```python
from build123d import *

# Parameters (mm, degrees)
SKETCH1_W           = 25.4
SKETCH1_H           = 25.4
SKETCH1_W_2         = 22.225
SKETCH1_H_2         = 22.225
BOSS_EXTRUDE1_DEPTH = 501.65
SKETCH4_R           = 6.35
CUT_EXTRUDE1_DEPTH  = 26.4
SKETCH5_R           = 1.5875
CUT_EXTRUDE2_DEPTH  = 26.4
SKETCH7_R           = 3.96875
CUT_EXTRUDE3_DEPTH  = 1.5875


with BuildPart() as part:
    # Sketch1 → Boss-Extrude1 (new body)
    with BuildSketch(Plane(origin=(0, 0, 0), x_dir=(1, 0, 0), z_dir=(0, 1, 0))):
        Rectangle(SKETCH1_W, SKETCH1_H)
        Rectangle(SKETCH1_W_2, SKETCH1_H_2, mode=Mode.SUBTRACT)
    extrude(amount=BOSS_EXTRUDE1_DEPTH)

    # Sketch4 → Cut-Extrude1 (cut, through all)
    with BuildSketch(Plane.XY.offset(12.7)):
        with Locations((0, 9.525)):
            Circle(SKETCH4_R)
    extrude(amount=-CUT_EXTRUDE1_DEPTH, mode=Mode.SUBTRACT)

    # Sketch5 → Cut-Extrude2 (cut, through all)
    with BuildSketch(Plane(origin=(0, 0, -12.7), x_dir=(-1, 0, 0), z_dir=(0, 0, -1))):
        with Locations((-5.709637497, 51.517813992)):
            Circle(SKETCH5_R)
        with Locations((5.709637497, 51.517813992)):
            Circle(SKETCH5_R)
    extrude(amount=-CUT_EXTRUDE2_DEPTH, mode=Mode.SUBTRACT)

    # Sketch7 → Cut-Extrude3 (cut)
    with BuildSketch(Plane.XY.offset(12.7)):
        with Locations((0, 30.5023012)):
            Circle(SKETCH7_R)
    extrude(amount=-CUT_EXTRUDE3_DEPTH, mode=Mode.SUBTRACT)


solid = part.part
```
Geometry: final body of the model. Coordinates: model frame, mm. A direction names the side the tool comes from. Round coordinates to 2 decimals unless told otherwise and drop trailing zeros. Loops run counter-clockwise (first coordinate to the right, second up) from the corner with the lowest first, then second, coordinate; pieces in that order, holes last.
Item 1: Contact query for flat-ended pins moving along their axis: P1, Ø1.9, axis at x = 5.71, y = 51.52, coming from the -Z side; P2, Ø5, axis at x = -2.5, z = 9.5, coming from the +Y side; P3, Ø5, axis at x = 0, y = 30.5, coming from the +Z side. Output: stop coordinate, or through.
Checked values:
P1: passes through
P2: stops at y = 501.65
P3: stops at z = -11.11
Item 2: Section C-C, the plane y = 303. Output: boundary loops of the cut face in (x, z).
Checked values:
outline: (-12.7, -12.7) - (12.7, -12.7) - (12.7, 12.7) - (-12.7, 12.7) - close; hole (-11.11, -11.11) - (11.11, -11.11) - (11.11, 11.11) - (-11.11, 11.11) - close
Item 3: Section A-A, the plane x = 0. State how many separate pieces and enclosed holes the cut face has, plus the area to 3 significant figures.
Checked values:
separate pieces: 5
enclosed holes: 0
area: 1,540 mm2
Item 4: Section B-B, the plane z = -6.75. Output: boundary loops of the cut face in (x, y).
Checked values:
outline: (-12.7, 0) - (-11.11, 0) - (-11.11, 501.65) - (-12.7, 501.65) - close; (11.11, 0) - (12.7, 0) - (12.7, 501.65) - (11.11, 501.65) - close
Item 5: Mould query, pull axis Y, two halves, no side actions, for faces 1 (the flat face through (-11.3, 501.65, -0.1)), 2 (the flat face through (0, 247, -12.7)), 3 (the cylindrical face through (-1.377, 3.326, -11.895)). Classes: released by +Y, released by -Y, zero draft, split by the parting line, or undercut.
Checked values:
face 1: released by +Y
face 2: zero draft
face 3: undercut
Item 6: Reachability of faces 4 (the flat face through (-11.3, 0, -0.1)), 5 (the cylindrical face through (-0.86, 26.628, 11.917)), 6 (the flat face through (-11.112, 247, 0)) from +Z, -Z, +X, -X, +Y, -Y: full face, straight path, thin tool, end or side. Return the list, or none.
Checked values:
face 4: +Z, -Z, +X, -X, -Y
face 5: +Z
face 6: +Y, -Y
Item 7: Line query: L1, parallel to Y at x = 0, z = -11.75 (3 decimals); L2, parallel to Z at x = -6.5, y = 340. Output: solid intervals per line, ascending.
Checked values:
L1: y = 0 to 3.175, 15.875 to 501.65
L2: z = -12.7 to -11.11, 11.11 to 12.7
